Read the model definition and answer for the solid it produces. Units are mm, in the model's axes. Face numbers are marked on the shaded views. Coordinates: 2 decimals unless noted, no trailing zeros. Loops run counter-clockwise (first coordinate to the right, second up) from the corner with the lowest first, then second, coordinate; pieces in that order, holes last. Notation, with made-up numbers: (11, 52.25) - (46, 52.25) arc R26 cw to (46, 81.25) - close; hole circle Ø6 at (-23.75, 25.5). An arc over 180 degrees is marked (long way). Use CSV: the item, a comma, the result in double quotes.
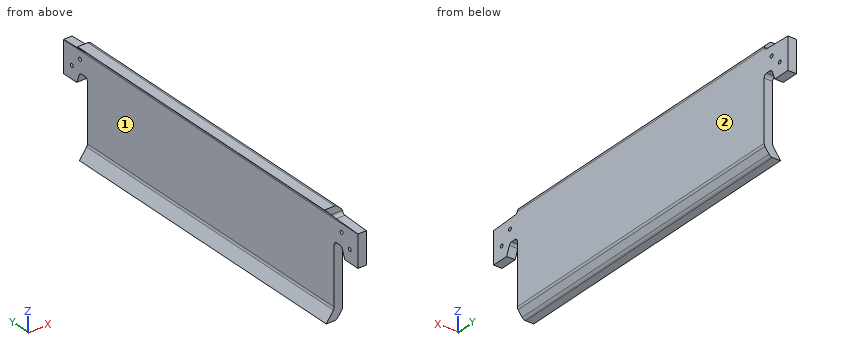
```python
from build123d import *

# Parameters (mm, degrees)
BOSS_EXTRUDE1_DEPTH = 95.885
BOSS_EXTRUDE2_DEPTH = 5.08
SKETCH5_R           = 1.0795
CUT_EXTRUDE1_DEPTH  = 130.08277933
FILLET2_R           = 1.905
FILLET3_R           = 2.54


with BuildPart() as part:
    # Sketch2 → Boss-Extrude1 (new, symmetric)
    with BuildSketch(Plane(origin=(0, 0, 0), x_dir=(1, 0, 0), z_dir=(0, 1, 0))):
        Polygon((0, 0), (-3.81, -3.81), (-10.994204897, -3.81), (-5.08, 2.104204897), (-5.08, 52.904204897), (-9.831464884, 59.69), (-3.629929973, 59.69), (0, 54.505922744), align=None)
    extrude(amount=BOSS_EXTRUDE1_DEPTH, both=True)

    # Sketch3 → Boss-Extrude2 (add)
    with BuildSketch(Plane.ZY.offset(5.08)):
        Polygon((-15.638409794, -95.885), (-15.638409794, -101.6), (-21.988409794, -104.14), (-21.988409794, -114.3), (-2.938409794, -114.3), (-2.104204897, -95.885), align=None)
        Polygon((-15.638409794, 95.885), (-2.104204897, 95.885), (-2.938409794, 114.3), (-21.988409794, 114.3), (-21.988409794, 104.14), (-15.638409794, 101.6), align=None)
    extrude(amount=-BOSS_EXTRUDE2_DEPTH)

    # Sketch5 → Cut-Extrude1 (cut, through all)
    with BuildSketch(Plane.ZY.offset(5.08)):
        with Locations((-40.64, -107.95)):
            Circle(SKETCH5_R)
        with Locations((-46.99, -101.6)):
            Circle(SKETCH5_R)
        with Locations((-46.99, 101.6)):
            Circle(SKETCH5_R)
        with Locations((-40.64, 107.95)):
            Circle(SKETCH5_R)
        with Locations((-8.018409794, -101.6)):
            Circle(SKETCH5_R)
        with Locations((-14.368409794, -107.95)):
            Circle(SKETCH5_R)
        with Locations((-8.018409794, 101.6)):
            Circle(SKETCH5_R)
        with Locations((-14.368409794, 107.95)):
            Circle(SKETCH5_R)
    extrude(amount=-CUT_EXTRUDE1_DEPTH, mode=Mode.SUBTRACT)

    # Fillet2
    # the kernel refuses this fillet: 1.905 mm, written as the material it adds along each edge
    with BuildSketch(Plane(origin=(-5.08, -95.885, -15.638409794), x_dir=(0, 0, -1), z_dir=(1, 0, 0))) as fillet2_piece_1:
        with BuildLine():
            CenterArc((FILLET2_R, -FILLET2_R), FILLET2_R, 90, 90)
            Line((0, -FILLET2_R), (0, 0))
            Line((0, 0), (FILLET2_R, 0))
        make_face()
    extrude(amount=5.08)
    with BuildSketch(Plane(origin=(-5.08, -95.885, -2.104204897), x_dir=(0, 0, 1), z_dir=(1, 0, 0))) as fillet2_piece_2_section:
        with BuildLine():
            CenterArc((FILLET2_R * 0.955725239349, FILLET2_R), FILLET2_R, 182.593742353, 87.406257647)
            Line((-FILLET2_R * 0.0432502788724, FILLET2_R * 0.954746116256), (0, 0))
            Line((0, 0), (FILLET2_R * 0.955725239349, 0))
        make_face()
    fillet2_piece_2 = extrude(amount=5.08, mode=Mode.PRIVATE)
    fillet2_piece_2 = split(fillet2_piece_2, bisect_by=Plane(origin=(-5.032232027, -97.010068738, -2.15197287), z_dir=(-0.7071067811865467, 0, -0.7071067811865485)), keep=Keep.TOP, mode=Mode.PRIVATE)
    add(fillet2_piece_2)
    with BuildSketch(Plane(origin=(-9.631641452, -95.885, -2.104204897), x_dir=(0, 0, 1), z_dir=(1, 0, 0))) as fillet2_piece_3_section:
        with BuildLine():
            CenterArc((FILLET2_R * 0.955725239349, FILLET2_R), FILLET2_R, 182.593742353, 87.406257647)
            Line((-FILLET2_R * 0.0432502788724, FILLET2_R * 0.954746116256), (0, 0))
            Line((0, 0), (FILLET2_R * 0.955725239349, 0))
        make_face()
    fillet2_piece_3 = extrude(amount=9.631641452, mode=Mode.PRIVATE)
    fillet2_piece_3 = split(fillet2_piece_3, bisect_by=Plane(origin=(-5.677063574, -96.058379599, -1.507141323), z_dir=(0.7071067811865467, 0, 0.7071067811865485)), keep=Keep.TOP, mode=Mode.PRIVATE)
    fillet2_piece_3 = split(fillet2_piece_3, bisect_by=Plane(origin=(-5.08, -96.058379599, -1.308120132), z_dir=(-1, 0, 0)), keep=Keep.TOP, mode=Mode.PRIVATE)
    add(fillet2_piece_3)
    with BuildSketch(Plane(origin=(-5.08, -95.885, -2.104204897), x_dir=(0, 0, 1), z_dir=(1, 0, 0))) as fillet2_piece_4_section:
        with BuildLine():
            CenterArc((FILLET2_R * 0.955725239349, FILLET2_R), FILLET2_R, 182.593742353, 87.406257647)
            Line((-FILLET2_R * 0.0432502788724, FILLET2_R * 0.954746116256), (0, 0))
            Line((0, 0), (FILLET2_R * 0.955725239349, 0))
        make_face()
    fillet2_piece_4 = extrude(amount=5.08, mode=Mode.PRIVATE)
    fillet2_piece_4 = split(fillet2_piece_4, bisect_by=Plane(origin=(-4.004458977, -96.293780551, -3.17974592), z_dir=(0.7071067811865467, 0, 0.7071067811865485)), keep=Keep.TOP, mode=Mode.PRIVATE)
    add(fillet2_piece_4)
    with BuildSketch(Plane(origin=(-5.08, -101.6, -15.638409794), x_dir=(0, 1, 0), z_dir=(1, 0, 0))) as fillet2_piece_5:
        with BuildLine():
            CenterArc((FILLET2_R * 0.677032961427, -FILLET2_R), FILLET2_R, 90, 68.198590514)
            Line((-FILLET2_R * 0.251443729458, -FILLET2_R * 0.628609323646), (0, 0))
            Line((0, 0), (FILLET2_R * 0.677032961427, 0))
        make_face()
    extrude(amount=5.08)
    with BuildSketch(Plane(origin=(-5.08, 95.885, -15.638409794), x_dir=(0, 0, -1), z_dir=(1, 0, 0))) as fillet2_piece_6:
        with BuildLine():
            CenterArc((FILLET2_R, FILLET2_R), FILLET2_R, 180, 90)
            Line((0, FILLET2_R), (0, 0))
            Line((0, 0), (FILLET2_R, 0))
        make_face()
    extrude(amount=5.08)
    with BuildSketch(Plane(origin=(-5.08, 101.6, -15.638409794), x_dir=(0, -1, 0), z_dir=(1, 0, 0))) as fillet2_piece_7:
        with BuildLine():
            CenterArc((FILLET2_R * 0.677032961427, FILLET2_R), FILLET2_R, 201.801409486, 68.198590514)
            Line((-FILLET2_R * 0.251443729458, FILLET2_R * 0.628609323646), (0, 0))
            Line((0, 0), (FILLET2_R * 0.677032961427, 0))
        make_face()
    extrude(amount=5.08)
    with BuildSketch(Plane(origin=(-5.08, 95.885, -2.104204897), x_dir=(0, 0, 1), z_dir=(1, 0, 0))) as fillet2_piece_8_section:
        with BuildLine():
            CenterArc((FILLET2_R * 0.955725239349, -FILLET2_R), FILLET2_R, 90, 87.406257647)
            Line((-FILLET2_R * 0.0432502788724, -FILLET2_R * 0.954746116256), (0, 0))
            Line((0, 0), (FILLET2_R * 0.955725239349, 0))
        make_face()
    fillet2_piece_8 = extrude(amount=5.08, mode=Mode.PRIVATE)
    fillet2_piece_8 = split(fillet2_piece_8, bisect_by=Plane(origin=(-5.032232027, 97.010068738, -2.15197287), z_dir=(-0.7071067811865467, 0, -0.7071067811865485)), keep=Keep.TOP, mode=Mode.PRIVATE)
    add(fillet2_piece_8)
    with BuildSketch(Plane(origin=(-9.631641452, 95.885, -2.104204897), x_dir=(0, 0, 1), z_dir=(1, 0, 0))) as fillet2_piece_9_section:
        with BuildLine():
            CenterArc((FILLET2_R * 0.955725239349, -FILLET2_R), FILLET2_R, 90, 87.406257647)
            Line((-FILLET2_R * 0.0432502788724, -FILLET2_R * 0.954746116256), (0, 0))
            Line((0, 0), (FILLET2_R * 0.955725239349, 0))
        make_face()
    fillet2_piece_9 = extrude(amount=9.631641452, mode=Mode.PRIVATE)
    fillet2_piece_9 = split(fillet2_piece_9, bisect_by=Plane(origin=(-5.677063574, 96.058379599, -1.507141323), z_dir=(0.7071067811865467, 0, 0.7071067811865485)), keep=Keep.TOP, mode=Mode.PRIVATE)
    fillet2_piece_9 = split(fillet2_piece_9, bisect_by=Plane(origin=(-5.08, 96.058379599, -1.308120132), z_dir=(-1, 0, 0)), keep=Keep.TOP, mode=Mode.PRIVATE)
    add(fillet2_piece_9)
    with BuildSketch(Plane(origin=(-5.08, 95.885, -2.104204897), x_dir=(0, 0, 1), z_dir=(1, 0, 0))) as fillet2_piece_10_section:
        with BuildLine():
            CenterArc((FILLET2_R * 0.955725239349, -FILLET2_R), FILLET2_R, 90, 87.406257647)
            Line((-FILLET2_R * 0.0432502788724, -FILLET2_R * 0.954746116256), (0, 0))
            Line((0, 0), (FILLET2_R * 0.955725239349, 0))
        make_face()
    fillet2_piece_10 = extrude(amount=5.08, mode=Mode.PRIVATE)
    fillet2_piece_10 = split(fillet2_piece_10, bisect_by=Plane(origin=(-4.004458977, 96.293780551, -3.17974592), z_dir=(0.7071067811865467, 0, 0.7071067811865485)), keep=Keep.TOP, mode=Mode.PRIVATE)
    add(fillet2_piece_10)

    # Fillet3
    fillet3_edges = [part.edges().sort_by_distance(p)[0] for p in [
        (-3.629929973, 0, -59.69),
        (-3.81, 0, 3.81),
        (0, 0, -54.505922744),
        (0, 0, 0),
        (-5.08, 0, -52.904204897),
        (-5.08, 0, -2.104204897),
    ]]
    fillet(fillet3_edges, radius=FILLET3_R)


solid = part.part
```
Q1. For a pull along Z with two mould halves and no side action, classify the marked faces 1 and 2 as +Z half, -Z half, draft (parallel to the pull), parting line (faces both ways), or undercut.
Reported:
face 1,"undercut"
face 2,"draft"
Q2. The part is cut by section B-B on y = 8. Determine the outline of the cut face in (x, z).
Reported:
outline,"(-10.99, 3.81) - (-5.82, -1.36) arc R2.54 cw to (-5.08, -3.16) - (-5.08, -52.1) arc R2.54 cw to (-5.54, -53.56) - (-9.83, -59.69) - (-4.95, -59.69) arc R2.54 ccw to (-2.87, -58.61) - (-0.46, -55.16) arc R2.54 ccw to (0, -53.71) - (0, -1.05) arc R2.54 ccw to (-0.74, 0.74) - (-3.07, 3.07) arc R2.54 ccw to (-4.86, 3.81) - close"
Q3. The part is cut by section C-C on z = -32.5. Determine the outline of the cut face in (x, y) (3 decimals), and give its area (3 significant figures).
Reported:
outline,"(-5.08, -95.885) - (0, -95.885) - (0, 95.885) - (-5.08, 95.885) - close"
area,"974 mm²"
Q4. The part is cut by section A-A on z = -20. Determine the outline of the cut face in (x, y) (3 decimals).
Reported:
outline,"(-5.08, -114.3) - (0, -114.3) - (0, -103.345) - (-5.08, -103.345) - close; (-5.08, -95.885) - (0, -95.885) - (0, 95.885) - (-5.08, 95.885) - close; (-5.08, 103.345) - (0, 103.345) - (0, 114.3) - (-5.08, 114.3) - close"
Q5. Given P1, Ø4.5, axis at x = -6, z = 2.5, coming from the +Y side (3 decimals); P2, Ø1.5, axis at x = -1.5, y = -107.5, coming from the -Z side; P3, Ø3.5, axis at y = -101.6, z = -8.02, coming from the +X side; P4, Ø3, axis at x = -3.5, y = -98.5, coming from the -Z side, each flat-ended and moving along its own axis, determine where each tip first touches the part or whether it passes through.
Reported:
P1,"stops at y = 95.885"
P2,"stops at z = -21.99"
P3,"stops at x = 0"
P4,"stops at z = -15.81"
Q6. Find the intervals of material crossed by probe 1 along Y at (x, z) = (-2.75, -7.5); probe 2 along X at (y, z) = (-79, -53); probe 3 along X at (y, z) = (21.5, -35), in increasing order. Write a range as [from, to].
Reported:
probe 1,"y = [-114.3, -102.55], [-100.65, 100.65], [102.55, 114.3]"
probe 2,"x = [-5.24, 0]"
probe 3,"x = [-5.08, 0]"
